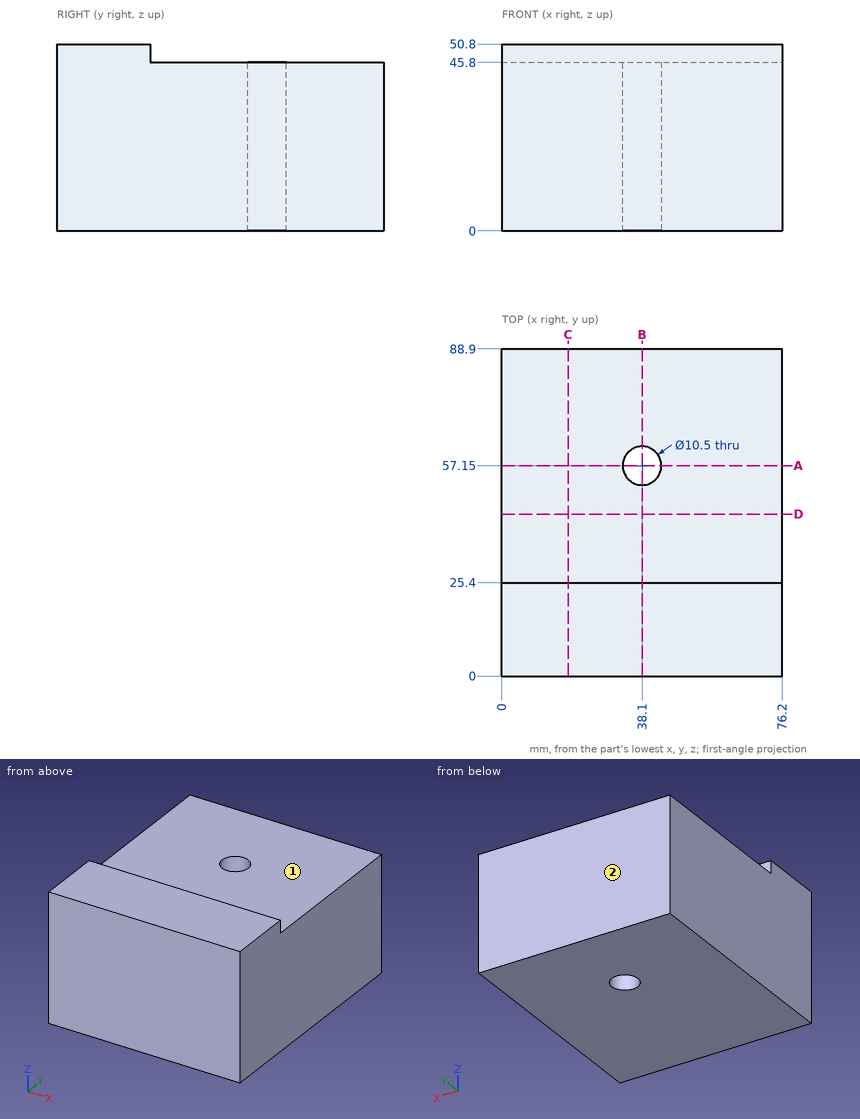
Here's the drawing with two shaded views (mm, measured from the low corner). I have some questions. A direction names the side the tool comes from. Coordinates: 2 decimals unless noted, no trailing zeros. Order: outer loops, then holes, each group sorted by start corner. A loop starts at its lowest first (then second) coordinate and runs counter-clockwise, first axis right, second up. Notation, with made-up numbers: M 75.25,1.25 L 81.25,1.25 A33 ccw 81.25,40.25 Z; hole C 25.5,80.5 d2. An arc over 180 degrees is marked long. Write item = value, one per line.
(1) I need wall thicknesses on line 1 along X through (y, z) = (57, 23); line 2 along Y through (x, z) = (38, 13); line 3 along Z through (x, y) = (16, 54). Which ranges of each line are inside material? Lowest first, please. Write a range as [from, to].
Results are:
line_1 = [0, 32.85], [43.35, 76.2]
line_2 = [0, 51.9], [62.4, 88.9]
line_3 = [0, 45.8]
(2) For pin 1 Ø8.5 at (x, y) = (38.1, 57.15) entering from +Z, with a flat end and sliding along its axis, tell me the tip position at first contact or that it passes through.
Results are:
pin_1 = through
(3) Suppose I cut it at C-C on x = 18. Please give me the cut outline in (y, z), plus the area to 3 significant figures.
Results are:
outline = M 0,0 L 88.9,0 L 88.9,45.8 L 25.4,45.8 L 25.4,50.8 L 0,50.8 Z
area = 4,200 mm2
(4) Suppose I cut it at B-B on x = 38.1. Please give me the cut outline in (y, z).
Results are:
outline = M 0,0 L 51.9,0 L 51.9,45.8 L 25.4,45.8 L 25.4,50.8 L 0,50.8 Z; M 62.4,0 L 88.9,0 L 88.9,45.8 L 62.4,45.8 Z
(5) Suppose I cut it at D-D on y = 44. Please give me the cut outline in (x, z).
Results are:
outline = M 0,0 L 76.2,0 L 76.2,45.8 L 0,45.8 Z
(6) Suppose I cut it at A-A on y = 57.15. Please give me the cut outline in (x, z).
Results are:
outline = M 0,0 L 32.85,0 L 32.85,45.8 L 0,45.8 Z; M 43.35,0 L 76.2,0 L 76.2,45.8 L 43.35,45.8 Z
(7) For the marked faces 1 and 2, which set-ups out of +Z, -Z, +X, -X, +Y, -Y let a thin tool reach every point of the face, with its end or its side?
Results are:
face_1 = +Z, +X, -X, +Y
face_2 = +Z, -Z, +X, -X, +Y
